Check sheet for the modelled part. Datum: model origin and axes. Units: mm. Face numbers are marked on the shaded views. A direction names the side the tool comes from. Give positions to 0.01 mm unless a question says otherwise; leave off trailing zeros. Write each loop counter-clockwise with the first axis right and the second up, starting at its lowest first coordinate (ties: lowest second). Pieces come first, ordered by that corner, then holes. Notation, with made-up numbers: (49, 62) -> (105, 62) arc R25 cw to (105, 74) -> close; hole circle Ø7 at (70.5, 59). An arc over 180 degrees is marked (long way). Return JSON: item names as keys, results as strings.
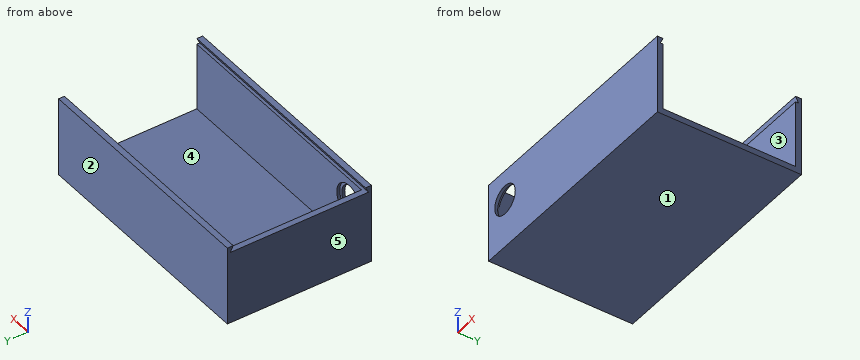
from build123d import *

# Parameters (mm, degrees)
F0_W           = 84.25
F0_H           = 49.28
F1_DEPTH       = 27.1
F2_W           = 80.25
F2_H           = 45.28
F3_DEPTH       = 25.1
F5_DEPTH       = 25
F5_DEPTH_BACK  = 25
F8_D           = 10
F8_DEPTH       = 2
F8_CBORE_D     = 12
F8_CBORE_DEPTH = 1
F9_W           = 4
F9_H           = 45.28
F10_DEPTH      = 2
F12_DEPTH      = 82.25
F13_W          = 49.28
F13_H          = 27.1
F13_W_2        = 18.18
F13_H_2        = 11.31
F14_DEPTH      = 2


with BuildPart() as f1:
    # F0 (on Top) → F1 (new body)
    with BuildSketch(Plane.XY):
        Rectangle(F0_W, F0_H)
    extrude(amount=F1_DEPTH)

    # F2 (on face) → F3 (cut)
    with BuildSketch(Plane.XY.offset(27.1)):
        Rectangle(F2_W, F2_H)
    extrude(amount=-F3_DEPTH, mode=Mode.SUBTRACT)

    # F4 (on face) → F5 (cut, two sides)
    with BuildSketch(Plane(origin=(40.125, 0, 0), x_dir=(0, -1, 0), z_dir=(-1, 0, 0))) as f5_sk:
        Polygon((-4.46, 20.205), (-22.64, 20.205), (-22.64, 14.55), (-22.64, 8.895), (-4.46, 8.895), align=None)
    extrude(amount=-F5_DEPTH, mode=Mode.SUBTRACT)
    extrude(f5_sk.sketch, amount=-F5_DEPTH_BACK, mode=Mode.SUBTRACT)

    # F8
    with Locations(Plane(origin=(0, -22.64, 0), x_dir=(-1, 0, 0), z_dir=(0, 1, 0))):
        with Locations((34.125, 16.76)):
            CounterBoreHole(F8_D / 2, F8_CBORE_D / 2, F8_CBORE_DEPTH, depth=F8_DEPTH)

    # F9 (on face) → F10 (cut)
    with BuildSketch(Plane.XY.offset(27.1)):
        with Locations((-40.125, 0)):
            Rectangle(F9_W, F9_H)
    extrude(amount=-F10_DEPTH, mode=Mode.SUBTRACT)

    # F11 (on face) → F12 (cut)
    with BuildSketch(Plane(origin=(-42.125, 0, 0), x_dir=(0, -1, 0), z_dir=(-1, 0, 0))):
        Polygon((22.64, 27.1), (22.64, 25.1), (23.64, 25.1), align=None)
        Polygon((-22.64, 27.1), (-23.64, 25.1), (-22.64, 25.1), align=None)
    extrude(amount=-F12_DEPTH, mode=Mode.SUBTRACT)

    # F13 (on face) → F14 (cut)
    with BuildSketch(Plane.YZ.offset(42.125)):
        with Locations((0, 13.55)):
            Rectangle(F13_W, F13_H)
        with Locations((13.55, 14.55)):
            Rectangle(F13_W_2, F13_H_2, mode=Mode.SUBTRACT)
    extrude(amount=-F14_DEPTH, mode=Mode.SUBTRACT)


solid = f1.part
(1) Cross-section at A-A on x = 10. Enter the section's corners in (y, z).
Reply:
{"outline": "(-24.64, 0) -> (24.64, 0) -> (24.64, 27.1) -> (22.64, 27.1) -> (23.64, 25.1) -> (22.64, 25.1) -> (22.64, 2) -> (-22.64, 2) -> (-22.64, 25.1) -> (-23.64, 25.1) -> (-22.64, 27.1) -> (-24.64, 27.1) -> close"}
(2) Thickness scan on L1, parallel to Y at x = 10.5, z = 22.5; L2, parallel to X at y = 16, z = 19.5 (3 decimals); L3, parallel to Z at x = -37.5, y = 6.5. Record the ranges inside material, lowest first.
Reply:
{"L1": "-24.64 to -22.64, 22.64 to 24.64", "L2": "-42.125 to -40.125", "L3": "0 to 2"}
(3) Cross-section at C-C on z = 14.5. Enter the section's corners in (x, y) (3 decimals).
Reply:
{"outline": "(-42.125, -24.64) -> (-38.585, -24.64) -> (-38.585, -23.64) -> (-39.683, -23.64) -> (-39.683, -22.64) -> (-40.125, -22.64) -> (-40.125, 22.64) -> (40.125, 22.64) -> (40.125, 24.64) -> (-42.125, 24.64) -> close; (-29.665, -24.64) -> (40.125, -24.64) -> (40.125, -22.64) -> (-28.567, -22.64) -> (-28.567, -23.64) -> (-29.665, -23.64) -> close"}
(4) Set-up check for the marked faces 4 and 5: record each of +Z, -Z, +X, -X, +Y, -Y from which the full face is reachable in a straight line by a thin tool's end or side.
Reply:
{"face 4": "+Z, +X", "face 5": "+Z, -Z, -X, +Y, -Y"}
(5) Depth check by flat-ended pin: pin 1 Ø1 at (x, y) = (-27.5, -18.5) entering from +Z; pin 2 Ø3 at (y, z) = (13.5, 19) entering from +X (3 decimals). Enter the tip coordinate at first touch or a pass-through.
Reply:
{"pin 1": "z = 2", "pin 2": "x = -40.125"}
(6) Cross-section at B-B on y = 14. Enter the section's corners in (x, z) (3 decimals).
Reply:
{"outline": "(-42.125, 0) -> (40.125, 0) -> (40.125, 2) -> (-40.125, 2) -> (-40.125, 25.1) -> (-42.125, 25.1) -> close"}
(7) Release check for a two-part mould opening along Y. For the marked faces 1, 2 and 3 record: pulls with the +Y half, pulls with the -Y half, needs draft (parallel to the pull), parting line crosses it, or undercut.
Reply:
{"face 1": "needs draft", "face 2": "pulls with the +Y half", "face 3": "undercut"}
